from build123d import *

# Parameters (mm, degrees)
F0_W     = 2
F0_H     = 40
F1_DEPTH = 42
F2_W     = 70
F2_H     = 40
F3_DEPTH = 2
F4_R     = 2


with BuildPart() as f1:
    # F0 (on Top) → F1 (new body)
    with BuildSketch(Plane.XY):
        Polygon((-37, 20), (-35, 20), (35, 20), (37, 20), (37, 22), (-37, 22), align=None)
        with Locations((-36, 0)):
            Rectangle(F0_W, F0_H)
        Polygon((35, -20), (-35, -20), (-37, -20), (-37, -22), (37, -22), (37, -20), align=None)
        with Locations((36, 0)):
            Rectangle(F0_W, F0_H)
    extrude(amount=F1_DEPTH)

    # F2 (on face) → F3 (join)
    with BuildSketch(Plane(origin=(0, 0, 0), x_dir=(1, 0, 0), z_dir=(0, 0, -1))):
        Rectangle(F2_W, F2_H)
    extrude(amount=-F3_DEPTH)

    # F4
    f4_edges = [f1.edges().sort_by_distance(p)[0] for p in [
        (37, -22, 21),
        (37, 22, 21),
        (-37, -22, 21),
        (-37, 22, 21),
    ]]
    fillet(f4_edges, radius=F4_R)


solid = f1.part
Here's how the part is built. I have some questions about the finished solid (model axes, mm). A direction names the side the tool comes from. Give positions to 0.01 mm unless a question says otherwise; leave off trailing zeros. Loops run counter-clockwise (first coordinate to the right, second up) from the corner with the lowest first, then second, coordinate; pieces in that order, holes last. Notation, with made-up numbers: (69, 79) -> (95, 79) arc R32 cw to (95, 107) -> close; hole circle Ø7 at (-9.5, -38.5). An arc over 180 degrees is marked (long way). Answer as a JSON object with one key per item and string values. Group by question number.
Item 1: Thinking about a two-plate mould opening in X: for faces 1 (the cylindrical face through (36.4, 21.43, 21.29)), 2 (the cylindrical face through (-36.4, 21.43, 21.29)), 3 (the flat face through (0, -20, 22)), 4 (the flat face through (0, 20, 22)), which applies, pulls with the +X half, pulls with the -X half, needs draft (parallel to the pull), parting line crosses it, or undercut?
Item 2: I need wall thicknesses on L1, parallel to Y at x = 9, z = 22; L2, parallel to X at y = -14, z = 11.5; L3, parallel to Z at x = 28, y = 6.5. Which ranges of each line are inside material? Lowest first, please.
Item 3: Imagine slicing it at B-B on x = 27. Write out the boundary of the cut face in (y, z), then the cut area to 3 significant figures.
Item 4: Will this pin go through, and if not, where does the flat tip stop? pin 1 (2 mm diameter, centred on x = -14.5, y = -5, fed in from +Z).
Item 5: Imagine slicing it at A-A on z = 13. Write out the boundary of the cut face in (x, y), then the cut area to 3 significant figures.
Item 6: Imagine slicing it at C-C on y = -16. Write out the boundary of the cut face in (x, z), then the cut area to 3 significant figures.
Item 7: On a 3-axis mill with a long thin cutter (end or side, diameter ignored), from which of +Z, -Z, +X, -X, +Y, -Y can I reach the whole of each face in a straight line? I mean faces 5 (the cylindrical face through (-36.43, -21.4, 21.29)), 6 (the flat face through (35, 0, 22)). Say none if no direction works.
Answer list:
{
 "1": {"face 1": "pulls with the +X half", "face 2": "pulls with the -X half", "face 3": "undercut", "face 4": "undercut"},
 "2": {"L1": "y = -22 to -20, 20 to 22", "L2": "x = -37 to -35, 35 to 37", "L3": "z = 0 to 2"},
 "3": {"outline": "(-22, 0) -> (22, 0) -> (22, 42) -> (20, 42) -> (20, 2) -> (-20, 2) -> (-20, 42) -> (-22, 42) -> close", "area": "248 mm2"},
 "4": {"pin 1": "stops at z = 2"},
 "5": {"outline": "(-37, -20) arc R2 ccw to (-35, -22) -> (35, -22) arc R2 ccw to (37, -20) -> (37, 20) arc R2 ccw to (35, 22) -> (-35, 22) arc R2 ccw to (-37, 20) -> close; hole (-35, -20) -> (35, -20) -> (35, 20) -> (-35, 20) -> close", "area": "453 mm2"},
 "6": {"outline": "(-37, 0) -> (37, 0) -> (37, 42) -> (35, 42) -> (35, 2) -> (-35, 2) -> (-35, 42) -> (-37, 42) -> close", "area": "308 mm2"},
 "7": {"face 5": "+Z, -Z, -X, -Y", "face 6": "+Z"}
}
